from build123d import *

# Parameters (mm, degrees)
SKETCH1_W                 = 25
SKETCH1_H                 = 15
SKETCH2_R                 = 12.7
BOSS_EXTRUDE1_DEPTH       = 3
SKETCH3_R                 = 22.4917
BOSS_EXTRUDE2_DEPTH       = 65.2
M6X1_0_TAPPED_HOLE1_D     = 5
M6X1_0_TAPPED_HOLE1_DEPTH = 10
M6X1_0_TAPPED_HOLE1_TIP   = 1.502151548
M6X1_0_TAPPED_HOLE2_D     = 5
M6X1_0_TAPPED_HOLE2_DEPTH = 15
M6X1_0_TAPPED_HOLE2_TIP   = 1.502151548


with BuildPart() as part:
    # Sketch1 → Revolve1 (revolve)
    with BuildSketch(Plane.XZ, mode=Mode.PRIVATE) as revolve1_sk:
        with Locations((12.5, 72.5)):
            Rectangle(SKETCH1_W, SKETCH1_H)
    revolve(revolve1_sk.sketch.rotate(Axis((0, 0, 80), (0, 0, -1)), 180), axis=Axis((0, 0, 80), (0, 0, -1)))

    # Sketch2 → Boss-Extrude1 (add)
    with BuildSketch(Plane.XY.offset(80)):
        Circle(SKETCH2_R)
    extrude(amount=BOSS_EXTRUDE1_DEPTH)

    # Sketch3 → Boss-Extrude2 (add)
    with BuildSketch(Plane(origin=(0, 0, 65), x_dir=(-1, 0, 0), z_dir=(0, 0, -1))):
        Circle(SKETCH3_R)
    extrude(amount=BOSS_EXTRUDE2_DEPTH)

    # M6x1.0 Tapped Hole1
    with Locations(Plane(origin=(0, 0, -0.2), x_dir=(-1, 0, 0), z_dir=(0, 0, -1))):
        with Locations((0, 17.5), (16.643489035, 5.407797402), (10.286241915, -14.157797402), (-10.286241915, -14.157797402), (-16.643489035, 5.407797402)):
            Hole(M6X1_0_TAPPED_HOLE1_D / 2, depth=M6X1_0_TAPPED_HOLE1_DEPTH)
            with Locations((0, 0, -(M6X1_0_TAPPED_HOLE1_DEPTH + M6X1_0_TAPPED_HOLE1_TIP / 2))):  # 118° drill point
                Cone(0, M6X1_0_TAPPED_HOLE1_D / 2, M6X1_0_TAPPED_HOLE1_TIP, mode=Mode.SUBTRACT)

    # M6x1.0 Tapped Hole2
    with Locations(Plane.XY.offset(80)):
        with Locations((-19.05, 0), (0, -19.05), (19.05, 0), (0, 19.05)):
            Hole(M6X1_0_TAPPED_HOLE2_D / 2, depth=M6X1_0_TAPPED_HOLE2_DEPTH)
            with Locations((0, 0, -(M6X1_0_TAPPED_HOLE2_DEPTH + M6X1_0_TAPPED_HOLE2_TIP / 2))):  # 118° drill point
                Cone(0, M6X1_0_TAPPED_HOLE2_D / 2, M6X1_0_TAPPED_HOLE2_TIP, mode=Mode.SUBTRACT)


solid = part.part
For this review, take the finished solid that the model builds, in its own axes (mm). A direction names the side the tool comes from. Give positions to 0.01 mm unless a question says otherwise; leave off trailing zeros. Order: outer loops, then holes, each group sorted by start corner. A loop starts at its lowest first (then second) coordinate and runs counter-clockwise, first axis right, second up. Notation, with made-up numbers: (-4, 37) - (51, 37) arc R20 cw to (51, 46) - close; hole circle Ø3 at (44, 14). An arc over 180 degrees is marked (long way). Answer as a JSON object with one key per item and string values. Group by question number.
Item 1: Clearance check with flat-ended pins moving along their axes: pin 1 Ø1 at (y, z) = (16, 60.5) entering from -X; pin 2 Ø8 at (y, z) = (-6.5, 35.5) entering from -X; pin 3 Ø6 at (x, y) = (0, -19.05) entering from +Z. State where each tip first meets the part, or that it passes through.
Item 2: Take a section at A-A on z = 75. Give the boundary of the cut face in (x, y).
Item 3: Wall thickness on line 1 along Y through (x, z) = (0, 75); line 2 along Z through (x, y) = (-18.5, -15); line 3 along Z through (x, y) = (11, 14.5): over which ranges is each line inside the solid? List them lowest first.
Item 4: Machinability: for faces 1 (the cylindrical face through (-1.15, 16.83, 72.4)), 2 (the cylindrical face through (-14.26, 6.16, 4.87)), 3 (the flat face through (0, 0, -0.2)), which of the approach directions +Z, -Z, +X, -X, +Y, -Y give a long, thin tool a straight path to every point of the face, cutting with its end or side? Answer none if there is none.
Item 5: Take a section at C-C on z = 43. Give the boundary of the cut face in (x, y).
Item 6: Take a section at B-B on x = 4. Give the boundary of the cut face in (y, z), and give its area (3 significant figures).
Item 7: Draft analysis for pull direction Y (two halves, no side actions). For faces 4 (the conical face through (0.4, -19.22, 63.76)), 5 (the cylindrical face through (-2.75, -12.4, 81.48)), 6 (the flat face through (-22.34, 3.82, 65)), state which applies: pulls with the +Y half, pulls with the -Y half, needs draft (parallel to the pull), parting line crosses it, or undercut.
Reported:
{
 "1": {"pin 1": "x = -16.3", "pin 2": "x = -22.35", "pin 3": "z = 80"},
 "2": {"outline": "circle Ø50 at (0, 0); hole circle Ø5 at (-19.05, 0); hole circle Ø5 at (0, -19.05); hole circle Ø5 at (0, 19.05); hole circle Ø5 at (19.05, 0)"},
 "3": {"line 1": "-25 to -21.55, -16.55 to 16.55, 21.55 to 25", "line 2": "65 to 80", "line 3": "-0.2 to 80"},
 "4": {"face 1": "+Z", "face 2": "-Z", "face 3": "-Z, +X, -X, +Y, -Y"},
 "5": {"outline": "circle Ø44.98 at (0, 0)"},
 "6": {"outline": "(-24.68, 65) - (-22.13, 65) - (-22.13, -0.2) - (22.13, -0.2) - (22.13, 65) - (24.68, 65) - (24.68, 80) - (12.05, 80) - (12.05, 83) - (-12.05, 83) - (-12.05, 80) - (-24.68, 80) - close", "area": "3,700 mm^2"},
 "7": {"face 4": "undercut", "face 5": "parting line crosses it", "face 6": "needs draft"}
}
